```python
from build123d import *

# Parameters (mm, degrees)
F1_DEPTH = 20


with BuildPart() as f1:
    # F0 (on Top) → F1 (new body)
    with BuildSketch(Plane.XY):
        with BuildLine():
            Line((20, -3.5), (20, 0))
            Line((20, 0), (0, 0))
            Line((0, 0), (0, 33.85))
            Line((0, 33.85), (20, 33.85))
            Line((20, 33.85), (20, 37.35))
            Line((20, 37.35), (-18.3, 37.35))
            Line((-18.3, 37.35), (-18.3, 36.186635))
            ThreePointArc((-18.3, 36.186635), (-17.266767, 33.142828), (-14.594095, 31.357006))
            Line((-14.594095, 31.357006), (-7.705905, 29.511321))
            ThreePointArc((-7.705905, 29.511321), (-5.033233, 27.725499), (-4, 24.681692))
            Line((-4, 24.681692), (-4, 16.925))
            Line((-4, 16.925), (-4, 9.168308))
            ThreePointArc((-4, 9.168308), (-5.033233, 6.124501), (-7.705905, 4.338679))
            Line((-7.705905, 4.338679), (-14.594095, 2.492994))
            ThreePointArc((-14.594095, 2.492994), (-17.266767, 0.707172), (-18.3, -2.336635))
            Line((-18.3, -2.336635), (-18.3, -3.5))
            Line((-18.3, -3.5), (20, -3.5))
        make_face()
    extrude(amount=F1_DEPTH)


solid = f1.part
```
Geometry check sheet. Reference: the model listing, model coordinates, mm. A direction names the side the tool comes from. Coordinates: 2 decimals unless noted, no trailing zeros. Order: outer loops, then holes, each group sorted by start corner. A loop starts at its lowest first (then second) coordinate and runs counter-clockwise, first axis right, second up. Notation, with made-up numbers: M -8.75,6.25 L 0.25,6.25 A27 ccw 0.25,34.25 Z; hole C -28.75,-10 d6. An arc over 180 degrees is marked long. Answer as a JSON object with one key per item and string values.
Q1. Cross-section at D-D on x = -5. Record the cut outline in (y, z).
Results are:
{"outline": "M -3.5,0 L 6.17,0 L 6.17,20 L -3.5,20 Z; M 27.68,0 L 37.35,0 L 37.35,20 L 27.68,20 Z"}
Q2. Cross-section at C-C on y = 22. Record the cut outline in (x, z), and give its area (3 significant figures).
Results are:
{"outline": "M -4,0 L 0,0 L 0,20 L -4,20 Z", "area": "80.0 mm²"}
Q3. Tool access check on faces 1 (the cylindrical face through (-17.294, 33.179, 9.86)), 2 (the flat face through (10, 0, 10)), 3 (the flat face through (-3, 19, 0)). Record the directions out of +Z, -Z, +X, -X, +Y, -Y that give a thin tool (end or side, any length) a straight path to the whole face; none if there is none.
Results are:
{"face 1": "+Z, -Z, -X", "face 2": "+Z, -Z, +X", "face 3": "-Z, +X, -X, +Y, -Y"}
Q4. Release check for a two-part mould opening along Y. For faces 4 (the flat face through (20, -2, 10)), 5 (the flat face through (1, -3.5, 10)), 6 (the flat face through (-4, 17, 10)), 7 (the flat face through (1, 37.35, 10)) record: released by +Y, released by -Y, zero draft, split by the parting line, or undercut.
Results are:
{"face 4": "zero draft", "face 5": "released by -Y", "face 6": "undercut", "face 7": "released by +Y"}
Q5. Scan lines: line 1 (Y direction, x = 6.5, z = 17); line 2 (X direction, y = 19, z = 7.75); line 3 (Y direction, x = -11, z = 10.25). Record each from-to range of solid material in increasing order.
Results are:
{"line 1": "y = -3.5 to 0, 33.85 to 37.35", "line 2": "x = -4 to 0", "line 3": "y = -3.5 to 3.46, 30.39 to 37.35"}
Q6. Cross-section at B-B on z = 11.25. Record the cut outline in (x, y), and give its area (3 significant figures).
Results are:
{"outline": "M -18.3,-3.5 L 20,-3.5 L 20,0 L 0,0 L 0,33.85 L 20,33.85 L 20,37.35 L -18.3,37.35 L -18.3,36.19 A5 ccw -14.59,31.36 L -7.71,29.51 A5 cw -4,24.68 L -4,9.17 A5 cw -7.71,4.34 L -14.59,2.49 A5 ccw -18.3,-2.34 Z", "area": "501 mm²"}
Q7. Cross-section at A-A on x = 6.5. Record the cut outline in (y, z).
Results are:
{"outline": "M -3.5,0 L 0,0 L 0,20 L -3.5,20 Z; M 33.85,0 L 37.35,0 L 37.35,20 L 33.85,20 Z"}
Q8. Depth check by flat-ended pin: pin 1 Ø6 at (y, z) = (11.5, 7.5) entering from +X; pin 2 Ø12 at (x, y) = (4, 29) entering from -Z; pin 3 Ø6 at (y, z) = (33, 3.5) entering from -X; pin 4 Ø8 at (y, z) = (20, 10.5) entering from -X. Enter the tip coordinate at first touch or a pass-through.
Results are:
{"pin 1": "stops at x = 0", "pin 2": "stops at z = 0", "pin 3": "stops at x = -18.3", "pin 4": "stops at x = -4"}
